Geometry check sheet. Reference: the model listing, model coordinates, mm. A direction names the side the tool comes from. Round coordinates to 2 decimals unless told otherwise and drop trailing zeros. Loops run counter-clockwise (first coordinate to the right, second up) from the corner with the lowest first, then second, coordinate; pieces in that order, holes last. Notation, with made-up numbers: (49, -37.75) - (86, -37.75) arc R31 cw to (86, -7.75) - close; hole circle Ø6 at (11.5, 70). An arc over 180 degrees is marked (long way). Write item = value, one per line.
```python
from build123d import *

# Parameters (mm, degrees)
F1_DEPTH      = 127
F2_W          = 95.25
F2_H          = 57.15
F3_DEPTH      = 83.3406583964
F4_R          = 2.54
F5_DEPTH      = 12.701
F6_R          = 2.54
F7_DEPTH      = 12.701
F8_W          = 106.045
F8_H          = 6.858
F8_W_2        = 10.795
F9_DEPTH      = 59.69
F10_W         = 95.25
F10_H         = 22.0760425496
F10_H_2       = 18.8356010627
F11_DEPTH     = 19.05
F12_W         = 119.38
F12_H         = 119.38
F12_R         = 6.35
F13_DEPTH     = 7.62
F14_T         = 5.08
F14_T3_DEPTH  = 17.78
F14_T5_DEPTH  = 26.035
F14_T7_DEPTH  = 29.21
F14_T9_DEPTH  = 105.41
F14_T11_DEPTH = 26.035
F14_T13_DEPTH = 17.1416638094
F14_T15_DEPTH = 43.2345651777
F14_T17_DEPTH = 16.002
F14_T19_DEPTH = 69.85
F14_T21_DEPTH = 127
F14_T23_DEPTH = 17.018
F14_T25_DEPTH = 17.018


# Not quite as in the source:
# - a shell that OpenCascade refuses in one call is made with other operations: the cavity is built on its own and cut out


with BuildPart() as f1:
    # F0 (on Right) → F1 (new body)
    with BuildSketch(Plane.YZ):
        with BuildLine():
            Line((0, 12.7), (0, 0))
            Line((0, 0), (127, 0))
            Line((127, 0), (127, 12.7))
            Line((127, 12.7), (98.9720369056, 12.7))
            Line((98.9720369056, 12.7), (98.9720369056, 80.0334606807))
            Line((98.9720369056, 80.0334606807), (107.95, 95.5837489087))
            Line((107.95, 95.5837489087), (91.4522160579, 105.1087489087))
            Line((91.4522160579, 105.1087489087), (88.9, 100.6881810245))
            Line((88.9, 100.6881810245), (41.7661742094, 19.05))
            ThreePointArc((41.7661742094, 19.05), (37.1176515813, 14.4014773719), (30.7676515813, 12.7))
            Line((30.7676515813, 12.7), (0, 12.7))
        make_face()
    extrude(amount=F1_DEPTH)

    # F2 (on face) → F3 (cut, through all)
    with BuildSketch(Plane(origin=(0, 23.075738686, -13.3227839421), x_dir=(1, 0, 0), z_dir=(0, -0.8660254038, 0.5))):
        with Locations((63.5, 108.1779547439)):
            Rectangle(F2_W, F2_H)
    extrude(amount=-F3_DEPTH, mode=Mode.SUBTRACT)

    # F4 (on face) → F5 (cut, through all)
    with BuildSketch(Plane.XY.offset(12.7)):
        with Locations((19.05, 12.7)):
            Circle(F4_R)
        with Locations((107.95, 12.7)):
            Circle(F4_R)
    extrude(amount=-F5_DEPTH, mode=Mode.SUBTRACT)

    # F6 (on face) → F7 (cut, through all)
    with BuildSketch(Plane.XY.offset(12.7)):
        with Locations((19.05, 114.3)):
            Circle(F6_R)
        with Locations((107.95, 114.3)):
            Circle(F6_R)
    extrude(amount=-F7_DEPTH, mode=Mode.SUBTRACT)

    # F8 (on face) → F9 (cut)
    with BuildSketch(Plane(origin=(0, 68.3764773719, 118.4315328508), x_dir=(1, 0, 0), z_dir=(0, 0.5, 0.8660254038))):
        with Locations((58.1025, 35.9165678842)):
            Rectangle(F8_W, F8_H)
        with Locations((116.5225, 35.9165678842)):
            Rectangle(F8_W_2, F8_H)
    extrude(amount=-F9_DEPTH, mode=Mode.SUBTRACT)

    # F10 (on face) → F11 (cut)
    with BuildSketch(Plane(origin=(0, 98.9720369056, 0), x_dir=(-1, 0, 0), z_dir=(0, 1, 0))):
        with Locations((-63.5, 23.7380212748)):
            Rectangle(F10_W, F10_H)
        with Locations((-63.5, 44.193843081)):
            Rectangle(F10_W, F10_H_2)
    extrude(amount=-F11_DEPTH, mode=Mode.SUBTRACT)

    # F12 (on face) → F13 (cut)
    with BuildSketch(Plane(origin=(0, 0, 0), x_dir=(1, 0, 0), z_dir=(0, 0, -1))):
        with Locations((63.5, -63.5)):
            Rectangle(F12_W, F12_H)
        with Locations((19.05, -114.3)):
            Circle(F12_R, mode=Mode.SUBTRACT)
        with Locations((107.95, -114.3)):
            Circle(F12_R, mode=Mode.SUBTRACT)
        with Locations((19.05, -12.7)):
            Circle(F12_R, mode=Mode.SUBTRACT)
        with Locations((107.95, -12.7)):
            Circle(F12_R, mode=Mode.SUBTRACT)
    extrude(amount=-F13_DEPTH, mode=Mode.SUBTRACT)

    # F14: shell of thickness 5.08, made by hand


with BuildPart() as f14_core1:
    # F14_t2: copy of F1
    add(f1.part)

    # the walls: a layer under each face that stays
    f14_faces = [f14_core1.faces().sort_by_distance(p)[0] for p in [
        (63.5, 0, 6.35),
        (63.5, 15.3838257906, 12.7),
        (125.4320987654, 107.15625, 0),
        (0, 63.5, 52.5543744543),
        (127, 63.5, 52.5543744543),
        (63.5, 37.1176515813, 14.4014773719),
        (105.41, 12.7, 6.35),
        (16.51, 12.7, 6.35),
        (63.5, 127, 6.35),
        (3.81, 63.5, 3.81),
        (63.5, 3.81, 3.81),
        (123.19, 63.5, 3.81),
        (63.5, 123.19, 3.81),
        (63.5, 103.4610184528, 12.7),
        (7.9375, 98.9720369056, 46.3667303403),
        (7.9375, 103.4610184528, 87.8086047947),
        (13.2291666667, 105.200369343, 97.1712489087),
        (105.8333333333, 50.0471811841, 33.3931248181),
        (119.0625, 98.9720369056, 46.3667303403),
        (119.0625, 103.4610184528, 87.8086047947),
        (124.3541666667, 105.200369343, 97.1712489087),
        (112.1833333333, 8.4666666667, 0),
        (23.2833333333, 8.4666666667, 0),
        (111.125, 90.912869343, 55.7293744543),
        (63.5, 79.9220369056, 29.2372825889),
        (15.875, 98.3301377958, 51.6049284688),
        (105.41, 114.3, 6.35),
        (16.51, 114.3, 6.35),
        (15.875, 79.6943762624, 78.9015729955),
        (13.4257142857, 68.7983221811, 54.1870537248),
        (5.08, 84.5586375764, 74.6267207327),
        (113.5742857143, 74.7375244003, 50.7580537248),
        (111.125, 79.6943762624, 78.9015729955),
        (63.5, 65.4068762624, 54.1548970824),
        (121.92, 84.5586375764, 74.6267207327),
        (101.6, 12.7, 3.81),
        (12.7, 12.7, 3.81),
        (12.7, 114.3, 3.81),
        (101.6, 114.3, 3.81),
        (63.5, 76.8988877958, 47.5199811301),
        (112.1833333333, 110.0666666667, 0),
        (23.2833333333, 110.0666666667, 0),
        (63.5, 69.6361375764, 48.7801925568),
    ]]
    thicken(f14_faces, amount=-F14_T, mode=Mode.SUBTRACT)

    # F14_s4 → F14_t3 (cut)
    with BuildSketch(Plane.XY.offset(-5.08)):
        Polygon((3.8608, 3.8608), (-1.27, 3.81), (-1.27, -1.27), (3.81, -1.27), align=None)
        Polygon((3.8608, 123.1392), (-1.27, 123.19), (-1.27, 128.27), (3.81, 128.27), align=None)
        Polygon((123.1392, 3.8608), (123.19, -1.27), (128.27, -1.27), (128.27, 3.81), align=None)
        Polygon((123.1392, 123.1392), (128.27, 123.19), (128.27, 128.27), (123.19, 128.27), align=None)
    extrude(amount=F14_T3_DEPTH, mode=Mode.SUBTRACT)

    # F14_s6 → F14_t5 (cut)
    with BuildSketch(Plane.YZ.offset(106.045)):
        Polygon((99.0228369056, 12.7508), (98.9720369056, 7.62), (93.8920369056, 7.62), (93.8920369056, 12.7), align=None)
        Polygon((99.0668309961, 80.0080606807), (93.8920369056, 80.0334606807), (93.8920369056, 81.3946425782), (94.5726278544, 82.5734606807), align=None)
    extrude(amount=F14_T5_DEPTH, mode=Mode.SUBTRACT)

    # F14_s8 → F14_t7 (cut)
    with BuildSketch(Plane.XZ.offset(-104.0520369056)):
        Polygon((111.0742, 12.7508), (111.125, 7.62), (116.205, 7.62), (116.205, 12.7), align=None)
        Polygon((15.9258, 12.7508), (15.875, 7.62), (10.795, 7.62), (10.795, 12.7), align=None)
    extrude(amount=F14_T7_DEPTH, mode=Mode.SUBTRACT)

    # F14_s10 → F14_t9 (cut)
    with BuildSketch(Plane.YZ.offset(10.795)):
        Polygon((79.9728369056, 12.7508), (79.9220369056, 7.62), (74.8420369056, 7.62), (74.8420369056, 12.7), align=None)
    extrude(amount=F14_T9_DEPTH, mode=Mode.SUBTRACT)

    # F14_s12 → F14_t11 (cut)
    with BuildSketch(Plane.YZ.offset(-5.08)):
        Polygon((99.0228369056, 12.7508), (98.9720369056, 7.62), (93.8920369056, 7.62), (93.8920369056, 12.7), align=None)
        Polygon((99.0668309961, 80.0080606807), (93.8920369056, 80.0334606807), (93.8920369056, 81.3946425782), (94.5726278544, 82.5734606807), align=None)
    extrude(amount=F14_T11_DEPTH, mode=Mode.SUBTRACT)

    # F14_s14 → F14_t13 (cut)
    with BuildSketch(Plane(origin=(0, 29.6748522628, -17.1327839421), x_dir=(1, 0, 0), z_dir=(0, 0.8660254038, -0.5))):
        Polygon((111.0742, -79.6537547439), (116.205, -79.6029547439), (116.205, -74.5229547439), (111.125, -74.5229547439), align=None)
        Polygon((15.9258, -79.6537547439), (10.795, -79.6029547439), (10.795, -74.5229547439), (15.875, -74.5229547439), align=None)
    extrude(amount=F14_T13_DEPTH, mode=Mode.SUBTRACT)

    # F14_s16 → F14_t15 (cut)
    with BuildSketch(Plane.XY.offset(7.62)):
        Polygon((111.0742, 79.9728369056), (116.205, 79.9220369056), (116.205, 74.8420369056), (111.125, 74.8420369056), align=None)
        Polygon((15.9258, 79.9728369056), (15.875, 74.8420369056), (10.795, 74.8420369056), (10.795, 79.9220369056), align=None)
    extrude(amount=F14_T15_DEPTH, mode=Mode.SUBTRACT)

    # F14_s18 → F14_t17 (cut)
    with BuildSketch(Plane(origin=(0, 18.6763296347, -10.7827839421), x_dir=(1, 0, 0), z_dir=(0, 0.8660254038, -0.5))):
        Polygon((15.9258, -79.6537547439), (10.795, -79.6029547439), (10.795, -74.5229547439), (15.875, -74.5229547439), align=None)
        Polygon((111.0742, -79.6537547439), (116.205, -79.6029547439), (116.205, -74.5229547439), (111.125, -74.5229547439), align=None)
    extrude(amount=F14_T17_DEPTH, mode=Mode.SUBTRACT)

    # F14_s20 → F14_t19 (cut)
    with BuildSketch(Plane(origin=(0, 70.9164773719, 122.830941902), x_dir=(1, 0, 0), z_dir=(0, -0.5, -0.8660254038))):
        Polygon((121.8692, -32.5383678842), (121.92, -27.4075678842), (127, -27.4075678842), (127, -32.4875678842), align=None)
        Polygon((5.1308, -32.5383678842), (5.08, -27.4075678842), (0, -27.4075678842), (0, -32.4875678842), align=None)
        Polygon((5.1308, -39.2947678842), (0, -39.3455678842), (0, -44.4255678842), (5.08, -44.4255678842), align=None)
        Polygon((121.8692, -39.2947678842), (121.92, -44.4255678842), (127, -44.4255678842), (127, -39.3455678842), align=None)
    extrude(amount=F14_T19_DEPTH, mode=Mode.SUBTRACT)

    # F14_s22 → F14_t21 (cut)
    with BuildSketch(Plane.YZ):
        Polygon((66.7359305573, 50.5132866473), (62.2671274156, 53.0346925568), (59.7271274156, 48.6352835056), (64.1265364668, 46.0952835056), align=None)
        Polygon((72.5871445955, 47.1350866473), (77.0051477372, 44.5256925568), (74.4651477372, 40.1262835056), (70.065738686, 42.6662835056), align=None)
    extrude(amount=F14_T21_DEPTH, mode=Mode.SUBTRACT)

    # F14_s24 → F14_t23 (cut)
    with BuildSketch(Plane(origin=(0, 38.4736703653, -22.2127839421), x_dir=(1, 0, 0), z_dir=(0, -0.8660254038, 0.5))):
        Polygon((5.1308, 77.1137547439), (0, 77.0629547439), (0, 71.9829547439), (5.08, 71.9829547439), align=None)
    extrude(amount=F14_T23_DEPTH, mode=Mode.SUBTRACT)

    # F14_s26 → F14_t25 (cut)
    with BuildSketch(Plane(origin=(0, 23.7356500437, -13.7037839421), x_dir=(1, 0, 0), z_dir=(0, 0.8660254038, -0.5))):
        Polygon((121.8692, -77.1137547439), (127, -77.0629547439), (127, -71.9829547439), (121.92, -71.9829547439), align=None)
    extrude(amount=F14_T25_DEPTH, mode=Mode.SUBTRACT)


with BuildPart() as f1_1:
    add(f1.part)

    # what is left inside the walls is the cavity
    f14_cavity = [f14_core1.part.solids().sort_by_distance(p)[0] for p in [
        (63.5, 72.850575, 7.6708),
    ]]
    add(f14_cavity, mode=Mode.SUBTRACT)


solid = f1_1.part
```
(1) Gauge pin test, flat ends, axial feed: pin 1 (6 mm diameter, centred on x = 52, z = 19, fed in from +Y); pin 2 (5 mm diameter, centred on y = 19, z = 12, fed in from -X); pin 3 (1.5 mm diameter, centred on x = 95.5, y = 87, fed in from +Z); pin 4 (8 mm diameter, centred on x = 85.5, y = 79, fed in from +Z). Record the tip position at first contact, or that the pin passes through.
Answers follow:
pin_1 = 79.92
pin_2 = 0
pin_3 = 12.7
pin_4 = 48.62
(2) Section check C-C (x = 58). Enter the section's corners in (y, z).
Answers follow:
outline = (0, 0) - (3.81, 0) - (3.81, 7.62) - (30.77, 7.62) arc R17.78 ccw to (46.17, 16.51) - (63.47, 46.48) - (74.47, 40.13) - (74.84, 40.78) - (74.84, 7.62) - (123.19, 7.62) - (123.19, 0) - (127, 0) - (127, 12.7) - (79.92, 12.7) - (79.92, 45.77) - (73.88, 49.27) - (72.61, 47.07) - (66.67, 50.49) - (67.94, 52.69) - (62.88, 55.62) - (41.77, 19.05) arc R12.7 cw to (30.77, 12.7) - (0, 12.7) - close
(3) Section check A-A (y = 114.3). Enter the section's corners in (x, z), then the cut area to 3 significant figures.
Answers follow:
outline = (0, 0) - (3.81, 0) - (3.81, 7.62) - (12.7, 7.62) - (12.7, 0) - (16.51, 0) - (16.51, 12.7) - (0, 12.7) - close; (21.59, 0) - (25.4, 0) - (25.4, 7.62) - (101.6, 7.62) - (101.6, 0) - (105.41, 0) - (105.41, 12.7) - (21.59, 12.7) - close; (110.49, 0) - (114.3, 0) - (114.3, 7.62) - (123.19, 7.62) - (123.19, 0) - (127, 0) - (127, 12.7) - (110.49, 12.7) - close
area = 768 mm²
(4) Section check B-B (z = 77). Enter the section's corners in (x, y) (3 decimals).
Answers follow:
outline = (0, 75.224) - (15.875, 75.224) - (15.875, 81.969) - (5.08, 81.969) - (5.08, 89.888) - (15.875, 89.888) - (15.875, 98.972) - (0, 98.972) - close; (111.125, 75.224) - (127, 75.224) - (127, 98.972) - (111.125, 98.972) - (111.125, 89.888) - (121.92, 89.888) - (121.92, 81.969) - (111.125, 81.969) - close
(5) Mould release check, pull along Z, two halves, no side actions. Record for faces 5 (the flat face through (63, 76, 7.62)), 6 (the flat face through (121.92, 76, 26)), 7 (the flat face through (8, 98.972, 46)), 8 (the flat face through (62.833, 76.857, 47.544)): pulls with the +Z half, pulls with the -Z half, needs draft (parallel to the pull), parting line crosses it, or undercut.
Answers follow:
face_5 = pulls with the -Z half
face_6 = needs draft
face_7 = undercut
face_8 = pulls with the +Z half
(6) Section check D-D (z = 33.5). Enter the section's corners in (x, y) (3 decimals), then the cut area to 3 significant figures.
Answers follow:
outline = (0, 50.109) - (127, 50.109) - (127, 98.972) - (111.125, 98.972) - (111.125, 79.922) - (15.875, 79.922) - (15.875, 98.972) - (0, 98.972) - close; hole (5.08, 55.975) - (121.92, 55.975) - (121.92, 93.892) - (116.205, 93.892) - (116.205, 74.842) - (10.795, 74.842) - (10.795, 93.892) - (5.08, 93.892) - close
area = 1,970 mm²
(7) Set-up check for faces 1 (the flat face through (15.875, 89, 45)), 2 (the flat face through (63, 16, 12.7)), 3 (the flat face through (8, 93.892, 40)), 4 (the flat face through (119, 98.972, 46)): record each of +Z, -Z, +X, -X, +Y, -Y from which the full face is reachable in a straight line by a thin tool's end or side.
Answers follow:
face_1 = +Z, +Y
face_2 = +Z, +X, -X, -Y
face_3 = -Z
face_4 = +X, -X, +Y
(8) Scan lines: L1, parallel to X at y = 114, z = 6; L2, parallel to X at y = 80, z = 22.5 (3 decimals); L3, parallel to Y at x = 107.95, z = 3.5. Record each from-to range of solid material in increasing order. Write a range as [from, to].
Answers follow:
L1 = [0, 3.81], [12.71, 16.53], [21.57, 25.39], [101.61, 105.43], [110.47, 114.29], [123.19, 127]
L2 = [0, 5.08], [10.795, 15.875], [111.125, 116.205], [121.92, 127]
L3 = [0, 3.81], [6.35, 10.16], [15.24, 19.05], [107.95, 111.76], [116.84, 120.65], [123.19, 127]
